The listing builds one solid part. Answer for the finished solid, in the listing's coordinates (mm). Face numbers are marked on the shaded views. Give positions to 0.01 mm unless a question says otherwise; leave off trailing zeros. Order: outer loops, then holes, each group sorted by start corner. A loop starts at its lowest first (then second) coordinate and runs counter-clockwise, first axis right, second up. Notation, with made-up numbers: (-34.75, 87) - (-17.75, 87) arc R18 ccw to (-17.75, 102) - close; hole circle Ø10 at (10.5, 56.5). An arc over 180 degrees is marked (long way). Answer in a Markdown table with one row per item.
from build123d import *

# Parameters (mm, degrees)
F1_DEPTH = 150
F2_R     = 0.99999


# Not quite as in the source:
# - a fillet or chamfer is up to 0.001 mm smaller than in the source, because OpenCascade refuses the exact size


with BuildPart() as f1:
    # F0 (on Top) → F1 (new body)
    with BuildSketch(Plane.XY):
        Polygon((29.2243703455, 8.5721745163), (29.2243703455, 6.1646732221), (34.1438145412, 2.8682211694), (35.2571452463, 4.5296948349), align=None)
        with BuildLine():
            ThreePointArc((-40.7756296545, -29.4393073201), (-40.1898432169, -30.8535208825), (-38.7756296545, -31.4393073201))
            Line((-38.7756296545, -31.4393073201), (37.2243703455, -31.4393073201))
            ThreePointArc((37.2243703455, -31.4393073201), (38.6385839078, -30.8535208825), (39.2243703455, -29.4393073201))
            Line((39.2243703455, -29.4393073201), (39.2243703455, 8.5606926799))
            Line((39.2243703455, 8.5606926799), (37.2243703455, 8.5606926799))
            Line((37.2243703455, 8.5606926799), (37.2243703455, -27.4393073201))
            ThreePointArc((37.2243703455, -27.4393073201), (36.6385839078, -28.8535208825), (35.2243703455, -29.4393073201))
            Line((35.2243703455, -29.4393073201), (29.2243703455, -29.4393073201))
            Line((29.2243703455, -29.4393073201), (29.2243703455, 6.1646732221))
            Line((29.2243703455, 6.1646732221), (29.2243703455, 8.5721745163))
            Line((29.2243703455, 8.5721745163), (27.2243703455, 8.5721745163))
            Line((27.2243703455, 8.5721745163), (27.2243703455, -3.4278254837))
            Line((27.2243703455, -3.4278254837), (24.2243703455, -3.4278254837))
            Line((24.2243703455, -3.4278254837), (24.2243703455, -4.9278254837))
            Line((24.2243703455, -4.9278254837), (27.2243703455, -4.9278254837))
            Line((27.2243703455, -4.9278254837), (27.2243703455, -7.9278254837))
            Line((27.2243703455, -7.9278254837), (24.2243703455, -7.9278254837))
            Line((24.2243703455, -7.9278254837), (24.2243703455, -9.4278254837))
            Line((24.2243703455, -9.4278254837), (27.2243703455, -9.4278254837))
            Line((27.2243703455, -9.4278254837), (27.2243703455, -22.4393073201))
            Line((27.2243703455, -22.4393073201), (-15.2756296545, -22.4393073201))
            Line((-15.2756296545, -22.4393073201), (-15.2756296545, -17.9393073201))
            Line((-15.2756296545, -17.9393073201), (-18.7756296545, -17.9393073201))
            Line((-18.7756296545, -17.9393073201), (-18.7756296545, -19.4393073201))
            Line((-18.7756296545, -19.4393073201), (-16.7756296545, -19.4393073201))
            Line((-16.7756296545, -19.4393073201), (-16.7756296545, -22.4393073201))
            Line((-16.7756296545, -22.4393073201), (-28.7756296545, -22.4393073201))
            Line((-28.7756296545, -22.4393073201), (-28.7756296545, -19.4393073201))
            Line((-28.7756296545, -19.4393073201), (-26.7756296545, -19.4393073201))
            Line((-26.7756296545, -19.4393073201), (-26.7756296545, -17.9393073201))
            Line((-26.7756296545, -17.9393073201), (-28.7756296545, -17.9393073201))
            Line((-28.7756296545, -17.9393073201), (-28.7756296545, -9.4278254837))
            Line((-28.7756296545, -9.4278254837), (-25.7756296545, -9.4278254837))
            Line((-25.7756296545, -9.4278254837), (-25.7756296545, -7.9278254837))
            Line((-25.7756296545, -7.9278254837), (-28.7756296545, -7.9278254837))
            Line((-28.7756296545, -7.9278254837), (-28.7756296545, -4.9278254837))
            Line((-28.7756296545, -4.9278254837), (-25.7756296545, -4.9278254837))
            Line((-25.7756296545, -4.9278254837), (-25.7756296545, -3.4278254837))
            Line((-25.7756296545, -3.4278254837), (-28.7756296545, -3.4278254837))
            Line((-28.7756296545, -3.4278254837), (-28.7756296545, 8.5721745163))
            Line((-28.7756296545, 8.5721745163), (-30.7756296545, 8.5721745163))
            Line((-30.7756296545, 8.5721745163), (-30.7756296545, -29.4393073201))
            Line((-30.7756296545, -29.4393073201), (-36.7756296545, -29.4393073201))
            ThreePointArc((-36.7756296545, -29.4393073201), (-38.1898432169, -28.8535208825), (-38.7756296545, -27.4393073201))
            Line((-38.7756296545, -27.4393073201), (-38.7756296545, 8.5606926799))
            Line((-38.7756296545, 8.5606926799), (-40.7756296545, 8.5606926799))
            Line((-40.7756296545, 8.5606926799), (-40.7756296545, -29.4393073201))
        make_face()
        Polygon((-28.7756296545, -24.4393073201), (27.2243703455, -24.4393073201), (27.2243703455, -29.4393073201), (-15.2756296545, -29.4393073201), (-16.7756296545, -29.4393073201), (-28.7756296545, -29.4393073201), (-28.7756296545, -26.4393073201), (-28.7756296545, -24.9393073201), align=None, mode=Mode.SUBTRACT)
    extrude(amount=F1_DEPTH)

    # F2 (radius 1 in the source; OpenCascade refuses exactly that, so slightly less here)
    f2_edges = [f1.edges().sort_by_distance(p)[0] for p in [
        (-40.77563, 8.560693, 75),
        (-38.77563, 8.560693, 75),
        (-30.77563, 8.572175, 75),
        (-28.77563, 8.572175, 75),
        (27.22437, 8.572175, 75),
        (29.22437, 8.572175, 75),
        (35.257145, 4.529695, 75),
        (34.143815, 2.868221, 75),
        (37.22437, 8.560693, 75),
        (39.22437, 8.560693, 75),
    ]]
    fillet(f2_edges, radius=F2_R)


solid = f1.part
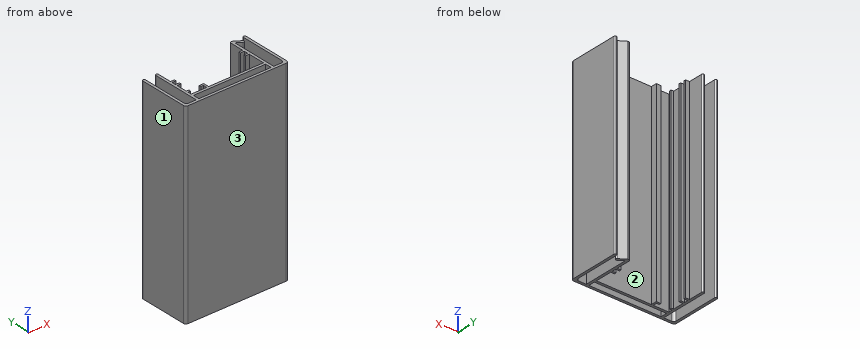
Item 1: Find section A-A on y = -16.5. Write down the section's boundary in (x, z).
Answer block:
| item | result |
|---|---|
| outline | (-40.78, 0) - (-38.78, 0) - (-38.78, 150) - (-40.78, 150) - close; (-30.78, 0) - (-28.78, 0) - (-28.78, 150) - (-30.78, 150) - close; (27.22, 0) - (29.22, 0) - (29.22, 150) - (27.22, 150) - close; (37.22, 0) - (39.22, 0) - (39.22, 150) - (37.22, 150) - close |
Item 2: Each of these flat-tipped pins is pushed along its axis until it touches: P1, Ø1.5, axis at x = -27.5, z = 88.5, coming from the +Y side; P2, Ø4, axis at x = -16.5, z = 88.5, coming from the +Y side; P3, Ø3, axis at x = -23, z = 89, coming from the +Y side. Where does it stop, or does it pass through?
Answer block:
| item | result |
|---|---|
| P1 | y = -3.43 |
| P2 | y = -17.94 |
| P3 | y = -22.44 |
Item 3: Consider line 1 (X direction, y = -22, z = 104); line 2 (X direction, y = -25, z = 30.5); line 3 (X direction, y = -24, z = 62.5). Determine where each line is inside the solid, lowest interval first.
Answer block:
| item | result |
|---|---|
| line 1 | -40.78 to -38.78, -30.78 to -28.78, -16.78 to -15.28, 27.22 to 29.22, 37.22 to 39.22 |
| line 2 | -40.78 to -38.78, -30.78 to -28.78, 27.22 to 29.22, 37.22 to 39.22 |
| line 3 | -40.78 to -38.78, -30.78 to 29.22, 37.22 to 39.22 |
Item 4: Determine the mould class of the marked faces 1, 2 and 3 for opening direction X: pulls with the +X half, pulls with the -X half, needs draft (parallel to the pull), parting line crosses it, or undercut.
Answer block:
| item | result |
|---|---|
| face 1 | pulls with the -X half |
| face 2 | undercut |
| face 3 | needs draft |
Item 5: Find section C-C on x = -33.5. Write down the section's boundary in (y, z).
Answer block:
| item | result |
|---|---|
| outline | (-31.44, 0) - (-29.44, 0) - (-29.44, 150) - (-31.44, 150) - close |
Item 6: Find section B-B on x = -5. Write down the section's boundary in (y, z).
Answer block:
| item | result |
|---|---|
| outline | (-31.44, 0) - (-29.44, 0) - (-29.44, 150) - (-31.44, 150) - close; (-24.44, 0) - (-22.44, 0) - (-22.44, 150) - (-24.44, 150) - close |
